```python
from build123d import *

# Parameters (mm, degrees)
SKETCH_R        = 7.5
PAD_DEPTH       = 10
SKETCH001_W     = 5
SKETCH001_H     = 11
POCKET_DEPTH    = 2
SKETCH002_R     = 5
POCKET001_DEPTH = 2


with BuildPart() as part:
    # Sketch → Pad (new body)
    with BuildSketch(Plane.XY):
        Circle(SKETCH_R)
    extrude(amount=PAD_DEPTH)

    # Sketch001 (on Face2 of Pad) → Pocket (cut)
    with BuildSketch(Plane(origin=(0, 0, 0), x_dir=(1, 0, 0), z_dir=(0, 0, -1))):
        Rectangle(SKETCH001_W, SKETCH001_H)
    extrude(amount=-POCKET_DEPTH, mode=Mode.SUBTRACT)

    # Sketch002 (on Face3 of Pocket) → Pocket001 (cut)
    with BuildSketch(Plane.XY.offset(10)):
        Circle(SKETCH002_R)
    extrude(amount=-POCKET001_DEPTH, mode=Mode.SUBTRACT)


solid = part.part
```
Verification items for the finished model (mm, model axes). A direction names the side the tool comes from. Coordinates: 2 decimals unless noted, no trailing zeros. Order: outer loops, then holes, each group sorted by start corner. A loop starts at its lowest first (then second) coordinate and runs counter-clockwise, first axis right, second up. Notation, with made-up numbers: (19, 69.25) -> (69, 69.25) arc R23 ccw to (69, 89.25) -> close; hole circle Ø5 at (66, 9). An arc over 180 degrees is marked (long way). Put each result on its own line as item: value. Start each with the question number.
1) Release check for a two-part mould opening along X. For faces 1 (the cylindrical face through (-7.493, 0.33, 4.93)), 2 (the flat face through (0, 0, 8)), 3 (the flat face through (0, 5.5, 1)), 4 (the flat face through (2, -5, 10)) record: pulls with the +X half, pulls with the -X half, needs draft (parallel to the pull), parting line crosses it, or undercut.
2) Cross-section at B-B (x = 0). Enter the section's corners in (y, z), plus the area to 3 significant figures.
3) Cross-section at A-A (y = 0). Enter the section's corners in (x, z), plus the area to 3 significant figures.
4) Cross-section at C-C (z = 1). Enter the section's corners in (x, y).
5) Cross-section at D-D (z = 4.5). Enter the section's corners in (x, y).
6) Tool access check on faces 5 (the flat face through (-2.5, 0, 1)), 6 (the cylindrical face through (-1.08, -4.88, 9.01)), 7 (the flat face through (3, 0, 0)). Record the directions out of +Z, -Z, +X, -X, +Y, -Y that give a thin tool (end or side, any length) a straight path to the whole face; none if there is none.
7) Material ranges on L1, parallel to Y at x = 0, z = 9.2; L2, parallel to Z at x = -4, y = 0.5; L3, parallel to X at y = 2.25, z = 9.25, recorded low to high.
8) Go/stop test with flat-tipped pins: pin 1 (1.5 mm diameter, centred on y = -2.5, z = 4, fed in from +X); pin 2 (3 mm diameter, centred on x = 0.5, z = 8.5, fed in from +Y); pin 3 (3 mm diameter, centred on x = 2, y = -1.5, fed in from +Z); pin 4 (1 mm diameter, centred on y = 2.5, z = 0.5, fed in from +X). Record where each tip stops, or that it passes through.
Geometry check:
1. face 1: parting line crosses it
1. face 2: undercut
1. face 3: undercut
1. face 4: needs draft
2. outline: (-7.5, 0) -> (-5.5, 0) -> (-5.5, 2) -> (5.5, 2) -> (5.5, 0) -> (7.5, 0) -> (7.5, 10) -> (5, 10) -> (5, 8) -> (-5, 8) -> (-5, 10) -> (-7.5, 10) -> close
2. area: 108 mm^2
3. outline: (-7.5, 0) -> (-2.5, 0) -> (-2.5, 2) -> (2.5, 2) -> (2.5, 0) -> (7.5, 0) -> (7.5, 10) -> (5, 10) -> (5, 8) -> (-5, 8) -> (-5, 10) -> (-7.5, 10) -> close
3. area: 120 mm^2
4. outline: circle Ø15 at (0, 0); hole (-2.5, -5.5) -> (2.5, -5.5) -> (2.5, 5.5) -> (-2.5, 5.5) -> close
5. outline: circle Ø15 at (0, 0)
6. face 5: -Z
6. face 6: +Z
6. face 7: -Z, +X, -X, +Y, -Y
7. L1: y = -7.5 to -5, 5 to 7.5
7. L2: z = 0 to 8
7. L3: x = -7.15 to -4.47, 4.47 to 7.15
8. pin 1: stops at x = 7.29
8. pin 2: stops at y = 7.5
8. pin 3: stops at z = 8
8. pin 4: stops at x = 7.23
